from build123d import *

# Parameters (mm, degrees)
F0_R     = 1
F1_DEPTH = 100
F2_R     = 1
F3_DEPTH = 25


with BuildPart() as f1:
    # F0 (on Top) → F1 (new body)
    with BuildSketch(Plane.XY):
        Polygon((2.701523, -0.15526), (2.02005, 1.80048), (0.15526, 2.701523), (-1.80048, 2.02005), (-2.701523, 0.15526), (-2.02005, -1.80048), (-0.15526, -2.701523), (1.80048, -2.02005), align=None)
        Circle(F0_R, mode=Mode.SUBTRACT)
        Circle(F0_R)
    extrude(amount=F1_DEPTH)

    # F2
    f2_edges = [f1.edges().sort_by_distance(p)[0] for p in [
        (0.82261, -2.360787, 0),
        (2.251001, -1.087655, 0),
        (2.360787, 0.82261, 0),
        (1.087655, 2.251001, 0),
        (-0.82261, 2.360787, 0),
        (-2.251001, 1.087655, 0),
        (-2.360787, -0.82261, 0),
        (-1.087655, -2.251001, 0),
        (0.82261, -2.360787, 100),
        (2.251001, -1.087655, 100),
        (2.360787, 0.82261, 100),
        (1.087655, 2.251001, 100),
        (-0.82261, 2.360787, 100),
        (-2.251001, 1.087655, 100),
        (-2.360787, -0.82261, 100),
        (-1.087655, -2.251001, 100),
    ]]
    fillet(f2_edges, radius=F2_R)

    # F0 (on Top) → F3 (cut)
    with BuildSketch(Plane.XY):
        Circle(F0_R)
    extrude(amount=F3_DEPTH, mode=Mode.SUBTRACT)


solid = f1.part
Design review of the part built by this model. Coordinates are the model's own, in mm. A direction names the side the tool comes from. Coordinates: 2 decimals unless noted, no trailing zeros. Loops run counter-clockwise (first coordinate to the right, second up) from the corner with the lowest first, then second, coordinate; pieces in that order, holes last. Notation, with made-up numbers: (50, 68.25) - (100, 68.25) arc R21 cw to (100, 85.25) - close; hole circle Ø5 at (35.5, 78). An arc over 180 degrees is marked (long way). Use CSV: the item, a comma, the result in double quotes. Start each with the question number.
1. To check wall thickness, follow probe 1 along Z at (x, y) = (-0.75, -0.6); probe 2 along Y at (x, z) = (2, 64.5); probe 3 along Y at (x, z) = (0.9, 21.5). State the ranges of each line that lie inside material, in increasing order.
2. Mouldability with a two-part tool opening along X and no side actions: class faces 1 (the cylindrical face through (0, -1, 12)), 2 (the flat face through (-0.809, 2.366, 49.314)), 3 (the flat face through (0, 0, 100)), 4 (the cylindrical face through (0.95, 2, 99.7)) as released by +X, released by -X, zero draft, split by the parting line, or undercut.
3. Clearance check with a flat-ended pin moving along its axis: pin 1 (2 mm diameter, centred on x = -1, z = 53.5, fed in from +Y). State where the tip first meets the part, or that it passes through.
4. Add section A-A on z = 56.5. Give the boundary of the cut face in (x, y).
5. For faces 5 (the flat face through (2.245, -1.101, 49.314)), 6 (the flat face through (0, 0, 25)), list the 3-axis set-ups (+Z, -Z, +X, -X, +Y, -Y) from which the entire face can be reached by the end or side of a thin tool; tool diameter is ignored.
Resolved:
1,probe 1,"25 to 100"
1,probe 2,"-1.61 to 1.81"
1,probe 3,"-2.33 to -0.44, 0.44 to 2.34"
2,face 1,"undercut"
2,face 2,"released by -X"
2,face 3,"zero draft"
2,face 4,"released by +X"
3,pin 1,"y = 2.65"
4,outline,"(-2.7, 0.16) - (-2.02, -1.8) - (-0.16, -2.7) - (1.8, -2.02) - (2.7, -0.16) - (2.02, 1.8) - (0.16, 2.7) - (-1.8, 2.02) - close"
5,face 5,"+Z, -Z, +X, -Y"
5,face 6,"-Z"
